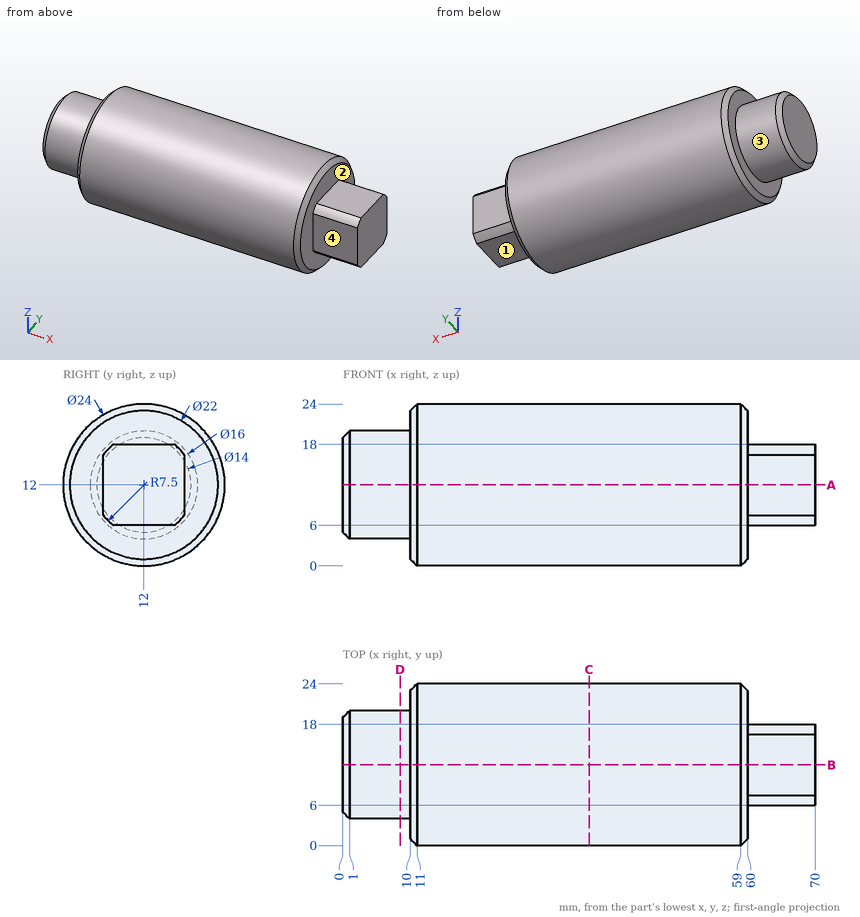
Part print with two shaded views. Sizes in mm from the minimum x, y, z corner. A direction names the side the tool comes from. Round coordinates to 2 decimals unless told otherwise and drop trailing zeros. Loops run counter-clockwise (first coordinate to the right, second up) from the corner with the lowest first, then second, coordinate; pieces in that order, holes last. Notation, with made-up numbers: (77, 27.25) - (94, 27.25) arc R13 cw to (94, 38.25) - close; hole circle Ø2 at (60.25, 36). An arc over 180 degrees is marked (long way). Answer as a JSON object with one key per item and string values.
Item 1: Wall check: L1, parallel to X at y = 19.25, z = 18.75; L2, parallel to Z at x = 63, y = 13.25. Give the ranges that are in metal, low to high.
Output:
{"L1": "10 to 60", "L2": "6 to 18"}
Item 2: Band-saw the part on A-A on z = 12. List the corners of the cut face in (x, y).
Output:
{"outline": "(0, 5) - (1, 4) - (10, 4) - (10, 1) - (11, 0) - (59, 0) - (60, 1) - (60, 6) - (70, 6) - (70, 18) - (60, 18) - (60, 23) - (59, 24) - (11, 24) - (10, 23) - (10, 20) - (1, 20) - (0, 19) - close"}
Item 3: Band-saw the part on C-C on x = 36.5. List the corners of the cut face in (y, z).
Output:
{"outline": "circle Ø24 at (12, 12)"}
Item 4: Pin check, flat tips, straight feed: pin 1 (5 mm diameter, centred on x = 26, y = 19, fed in from +Z); pin 2 (2.5 mm diameter, centred on x = 67, y = 10, fed in from +Z); pin 3 (4 mm diameter, centred on x = 27.5, z = 3.5, fed in from -Y). Stop position of each tip, or through.
Output:
{"pin 1": "z = 23.12", "pin 2": "z = 18", "pin 3": "y = 1.91"}
Item 5: Tool access for the marked faces 1, 2, 3 and 4: list every direction of +Z, -Z, +X, -X, +Y, -Y with a clear straight run to the whole face (end or side of a thin tool).
Output:
{"face 1": "-Z, +X, +Y, -Y", "face 2": "+X", "face 3": "-X", "face 4": "+Z, -Z, +X, -Y"}
Item 6: Band-saw the part on D-D on x = 8.5. List the corners of the cut face in (y, z), plus the area to 3 significant figures.
Output:
{"outline": "circle Ø16 at (12, 12)", "area": "201 mm2"}
